```python
from build123d import *

# Parameters (mm, degrees)
F1_DEPTH      = 12
F1_DEPTH_BACK = 3
F2_DEPTH      = 12
F2_DEPTH_BACK = 3
F3_T1_DEPTH   = 15.504504139
F3_T3_DEPTH   = 15.504504139
F4_R          = 1
F5_DEPTH      = 5


# Not quite as in the source:
# - a fillet or chamfer that OpenCascade refuses, or shapes differently, is made with other operations: its cross-section is extruded or revolved along the edge and cut away or added


with BuildPart() as f1:
    # F0 (on Front) → F1 (new body, two sides)
    with BuildSketch(Plane.XZ) as f1_sk:
        with BuildLine():
            Line((10, -6.2486935191), (8.4804809616, -5.2991926423))
            ThreePointArc((8.4804809616, -5.2991926423), (4.8480962025, -8.7461970714), (0, -10))
            Line((0, -10), (10, -10))
            Line((10, -10), (10, -6.2486935191))
        make_face()
        with BuildLine():
            Line((-10, -10), (0, -10))
            ThreePointArc((0, -10), (-4.8480962025, -8.7461970714), (-8.4804809616, -5.2991926423))
            Line((-8.4804809616, -5.2991926423), (-10, -6.2486935191))
            Line((-10, -6.2486935191), (-10, -10))
        make_face()
        with BuildLine():
            Line((8.4804809616, -5.2991926423), (7.2084088173, -4.504313746))
            ThreePointArc((7.2084088173, -4.504313746), (4.1208817721, -7.4342675107), (0, -8.5))
            Line((0, -8.5), (0, -10))
            ThreePointArc((0, -10), (4.8480962025, -8.7461970714), (8.4804809616, -5.2991926423))
        make_face()
        with BuildLine():
            Line((0, -10), (0, -8.5))
            ThreePointArc((0, -8.5), (-4.1208817721, -7.4342675107), (-7.2084088173, -4.504313746))
            Line((-7.2084088173, -4.504313746), (-8.4804809616, -5.2991926423))
            ThreePointArc((-8.4804809616, -5.2991926423), (-4.8480962025, -8.7461970714), (0, -10))
        make_face()
        with BuildLine():
            ThreePointArc((-7.2084088173, -4.504313746), (-8.5, 0), (-7.2084088173, 4.504313746))
            Line((-7.2084088173, 4.504313746), (-8.4804809616, 5.2991926423))
            ThreePointArc((-8.4804809616, 5.2991926423), (-9.6126169594, 2.7563735582), (-10, 0))
            ThreePointArc((-10, 0), (-9.6126169594, -2.7563735582), (-8.4804809616, -5.2991926423))
            Line((-8.4804809616, -5.2991926423), (-7.2084088173, -4.504313746))
        make_face()
        with BuildLine():
            Line((-10, -6.2486935191), (-8.4804809616, -5.2991926423))
            ThreePointArc((-8.4804809616, -5.2991926423), (-9.6126169594, -2.7563735582), (-10, 0))
            Line((-10, 0), (-10, -6.2486935191))
        make_face()
    extrude(amount=F1_DEPTH)
    extrude(f1_sk.sketch, amount=-F1_DEPTH_BACK)

    # F0 (on Front) → F2 (join, two sides)
    with BuildSketch(Plane.XZ) as f2_sk:
        with BuildLine():
            Line((-10, -10), (0, -10))
            ThreePointArc((0, -10), (-4.8480962025, -8.7461970714), (-8.4804809616, -5.2991926423))
            Line((-8.4804809616, -5.2991926423), (-10, -6.2486935191))
            Line((-10, -6.2486935191), (-10, -10))
        make_face()
        with BuildLine():
            Line((8.4804809616, -5.2991926423), (7.2084088173, -4.504313746))
            ThreePointArc((7.2084088173, -4.504313746), (4.1208817721, -7.4342675107), (0, -8.5))
            Line((0, -8.5), (0, -10))
            ThreePointArc((0, -10), (4.8480962025, -8.7461970714), (8.4804809616, -5.2991926423))
        make_face()
        with BuildLine():
            Line((0, -10), (0, -8.5))
            ThreePointArc((0, -8.5), (-4.1208817721, -7.4342675107), (-7.2084088173, -4.504313746))
            Line((-7.2084088173, -4.504313746), (-8.4804809616, -5.2991926423))
            ThreePointArc((-8.4804809616, -5.2991926423), (-4.8480962025, -8.7461970714), (0, -10))
        make_face()
        with BuildLine():
            Line((10, -6.2486935191), (8.4804809616, -5.2991926423))
            ThreePointArc((8.4804809616, -5.2991926423), (4.8480962025, -8.7461970714), (0, -10))
            Line((0, -10), (10, -10))
            Line((10, -10), (10, -6.2486935191))
        make_face()
        with BuildLine():
            ThreePointArc((7.2084088173, 4.504313746), (8.1707244155, 2.3429175244), (8.5, 0))
            ThreePointArc((8.5, 0), (8.1707244155, -2.3429175244), (7.2084088173, -4.504313746))
            Line((7.2084088173, -4.504313746), (8.4804809616, -5.2991926423))
            ThreePointArc((8.4804809616, -5.2991926423), (9.6126169594, -2.7563735582), (10, 0))
            ThreePointArc((10, 0), (9.6126169594, 2.7563735582), (8.4804809616, 5.2991926423))
            Line((8.4804809616, 5.2991926423), (7.2084088173, 4.504313746))
        make_face()
        with BuildLine():
            ThreePointArc((10, 0), (9.6126169594, -2.7563735582), (8.4804809616, -5.2991926423))
            Line((8.4804809616, -5.2991926423), (10, -6.2486935191))
            Line((10, -6.2486935191), (10, 0))
        make_face()
    extrude(amount=-F2_DEPTH)
    extrude(f2_sk.sketch, amount=F2_DEPTH_BACK)

    # F3: fillet of radius 3 on 2 edges, made by hand

    # F3_s2 → F3_t1 (cut)
    with BuildSketch(Plane.XZ.offset(-18.504504139)):
        with BuildLine():
            ThreePointArc((-9.4148617579, -5.883058565), (-7.5407373956, -5.4407106546), (-5.783772496, -6.2288021091))
            ThreePointArc((-5.783772496, -6.2288021091), (-6.5530648439, -5.413625509), (-7.2084088173, -4.504313746))
            Line((-7.2084088173, -4.504313746), (-9.4148617579, -5.883058565))
        make_face()
    extrude(amount=F3_T1_DEPTH, mode=Mode.SUBTRACT)

    # F3_s4 → F3_t3 (cut)
    with BuildSketch(Plane.XZ.offset(3)):
        with BuildLine():
            ThreePointArc((5.783772496, -6.2288021091), (7.5407373956, -5.4407106546), (9.4148617579, -5.883058565))
            Line((9.4148617579, -5.883058565), (7.2084088173, -4.504313746))
            ThreePointArc((7.2084088173, -4.504313746), (6.5530648439, -5.413625509), (5.783772496, -6.2288021091))
        make_face()
    extrude(amount=F3_T3_DEPTH, mode=Mode.SUBTRACT)

    # F4
    f4_edges = [f1.edges().sort_by_distance(p)[0] for p in [
        (8.480481, 4.5, 5.299193),
        (-8.480481, -4.5, 5.299193),
    ]]
    fillet(f4_edges, radius=F4_R)

    # F5 (add): a face of the model
    f5_faces = [f1.faces().sort_by_distance(p)[0] for p in [
        (0, 0, -10),
    ]]
    extrude(f5_faces, amount=F5_DEPTH)


solid = f1.part
```
The model under review builds one solid part; all positions refer to its coordinate system, in mm. Round coordinates to 2 decimals unless told otherwise and drop trailing zeros. Loops run counter-clockwise (first coordinate to the right, second up) from the corner with the lowest first, then second, coordinate; pieces in that order, holes last. Notation, with made-up numbers: M 78.5,56 L 87.5,56 A20 cw 87.5,88 Z; hole C -20,31.5 d5. An arc over 180 degrees is marked long. Write item = value, one per line.
Item 1: Insertion check: P1, Ø4.5, axis at x = -7.5, z = -3, coming from the +Y side; P2, Ø1, axis at x = 7, z = 0.5, coming from the -Y side; P3, Ø2, axis at x = 7.5, z = 1.5, coming from the -Y side; P4, Ø4, axis at x = 2, y = -6, coming from the +Z side. Each pin has a flat end and moves straight along its axis. Give the tip position at first contact, or say it passes through.
Return value:
P1 = 3
P2 = through
P3 = -3
P4 = -7.5
Item 2: Take a section at D-D on y = -5. Write out the cut boundary in (x, z), then the cut area to 3 significant figures.
Return value:
outline = M -10,-15 L 10,-15 L 10,-6.25 L 9.41,-5.88 A3 ccw 5.78,-6.23 A8.5 cw -7.21,4.5 L -7.59,4.74 A1 ccw -9.02,4.32 A10 ccw -10,0 Z
area = 182 mm2
Item 3: Take a section at C-C on x = -2.25. Write out the cut boundary in (y, z).
Return value:
outline = M -12,-15 L 12,-15 L 12,-8.2 L -12,-8.2 Z
Item 4: For line 1 (X direction, y = -7, z = 0); line 2 (X direction, y = 0.5, z = -0.75); line 3 (X direction, y = 10, z = -5.75), list the stretches that pass through material, from the lowest coordinate up. Write a range as [from, to].
Return value:
line_1 = [-10, -8.5]
line_2 = [-10, -8.47], [8.47, 10]
line_3 = [-9.18, -6.47], [6.26, 10]
Item 5: The part is to be moulded in two halves that separate along X. For faces 1 (the cylindrical face through (9.758, 4.605, 2.187)), 2 (the cylindrical face through (7.513, -7.437, -5.443)), 3 (the cylindrical face through (-7.57, 7.56, -5.44)), 4 (the flat face through (2, 12, -9)), say which applies: released by +X, released by -X, zero draft, split by the parting line, or undercut.
Return value:
face_1 = released by +X
face_2 = undercut
face_3 = undercut
face_4 = zero draft
Item 6: Take a section at B-B on z = 2.25. Write out the cut boundary in (x, y), then the cut area to 3 significant figures.
Return value:
outline = M -9.74,-12 L -8.2,-12 L -8.2,3 L -9.74,3 Z; M 8.2,-3 L 9.74,-3 L 9.74,12 L 8.2,12 Z
area = 46.4 mm2
Item 7: Take a section at A-A on y = -2. Write out the cut boundary in (x, z), then the cut area to 3 significant figures.
Return value:
outline = M -10,-15 L 10,-15 L 10,0 A10 ccw 9.02,4.32 A1 ccw 7.59,4.74 L 7.21,4.5 A8.5 cw long -7.21,4.5 L -7.59,4.74 A1 ccw -9.02,4.32 A10 ccw -10,0 Z
area = 202 mm2
